Can you work these out from the model? Positions are in its coordinate system, mm. Round coordinates to 2 decimals unless told otherwise and drop trailing zeros. Loops run counter-clockwise (first coordinate to the right, second up) from the corner with the lowest first, then second, coordinate; pieces in that order, holes last. Notation, with made-up numbers: (11, 65) -> (23, 65) arc R22 ccw to (23, 83) -> close; hole circle Ø6 at (88.25, -27). An arc over 180 degrees is marked (long way). Use a Markdown table: item, result.
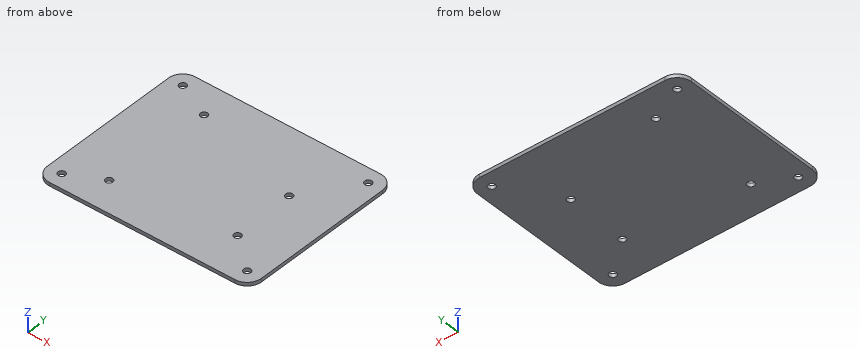
from build123d import *

# Parameters (mm, degrees)
F1_DEPTH = 1.5875
F2_D     = 3.175


with BuildPart() as f1:
    # F0 (on Top) → F1 (new body)
    with BuildSketch(Plane.XY):
        with BuildLine():
            ThreePointArc((0, 6.35), (1.859872, 1.859872), (6.35, 0))
            Line((6.35, 0), (88.9, 0))
            ThreePointArc((88.9, 0), (93.390128, 1.859872), (95.25, 6.35))
            Line((95.25, 6.35), (95.25, 69.85))
            ThreePointArc((95.25, 69.85), (93.390128, 74.340128), (88.9, 76.2))
            Line((88.9, 76.2), (6.35, 76.2))
            ThreePointArc((6.35, 76.2), (1.859872, 74.340128), (0, 69.85))
            Line((0, 69.85), (0, 6.35))
        make_face()
    extrude(amount=-F1_DEPTH)

    # F2 (through all)
    with Locations(Plane.XY):
        with Locations((6.35, 69.85), (22.290519, 62.23), (73.090519, 46.99), (88.9, 69.85), (88.9, 6.35), (73.848069, 19.05), (21.020519, 13.97), (6.35, 6.35)):
            Hole(F2_D / 2)


solid = f1.part
1. Will this pin go through, and if not, where does the flat tip stop? pin 1 Ø3 at (x, y) = (6.35, 6.35) entering from -Z.
Answer sheet:
| item | result |
|---|---|
| pin 1 | passes through |
2. I need wall thicknesses on line 1 (Y direction, x = 6.35, z = -0.75); line 2 (X direction, y = 69.85, z = -0.9); line 3 (X direction, y = 47, z = -0.45). Which ranges of each line are inside material? Lowest first, please.
Answer sheet:
| item | result |
|---|---|
| line 1 | y = 0 to 4.76, 7.94 to 68.26, 71.44 to 76.2 |
| line 2 | x = 0 to 4.76, 7.94 to 87.31, 90.49 to 95.25 |
| line 3 | x = 0 to 71.5, 74.68 to 95.25 |
3. I want a section at A-A (y = 62.23). Please give me the cut outline in (x, z), plus the area to 3 significant figures.
Answer sheet:
| item | result |
|---|---|
| outline | (0, -1.59) -> (20.7, -1.59) -> (20.7, 0) -> (0, 0) -> close; (23.88, -1.59) -> (95.25, -1.59) -> (95.25, 0) -> (23.88, 0) -> close |
| area | 146 mm² |
